Input: part model. Units: mm. Frame: model coordinates. Coordinates: 2 decimals unless noted, no trailing zeros. Loops run counter-clockwise (first coordinate to the right, second up) from the corner with the lowest first, then second, coordinate; pieces in that order, holes last.
Item 1: Section A-A on y = 0. Return loops of the section in (x, z), and give its area (3 significant figures).
Item 2: Contact query for a flat-ended pin moving along its axis: P1, Ø3, axis at x = -9.26, y = 19.87, coming from the +Z side. Output: stop coordinate, or through.
Item 3: Section B-B on x = 5. Return loops of the section in (y, z).
Item 4: Pull-direction query (Y, two-part tool) for faces 1 (the flat face through (-12, 27, 3)), 2 (the cylindrical face through (-21.156, -8.081, 1.521)), 3 (the cylindrical face through (-75.49, -45.72, 1.48)); classes: released by +Y, released by -Y, zero draft, split by the parting line, or undercut.
Item 5: Section C-C on z = 0.8. Give the number of separate pieces and of enclosed holes in the cut face, and give its area (3 significant figures).
Item 6: Ray query, line 1 along X through (y, z) = (89, 2.75); line 2 along Y through (x, z) = (-65, 2.15); line 3 along Y through (x, z) = (-67.5, 0.85). Return the intervals inside material, ascending.
```python
from build123d import *

# Parameters (mm, degrees)
BASE_FLANGE1_DEPTH   = 3
SKETCH2_R            = 15.5
SKETCH2_R_2          = 1.75
CUT_EXTRUDE1_DEPTH   = 131.05864062
M5_CLEARANCE_HOLE1_D = 5.5


# Sheet-metal steps are written as plain solids
with BuildPart() as part:
    # Sketch1 → Base-Flange1 (new body)
    with BuildSketch(Plane.XY):
        with BuildLine():
            Line((-67.5, 102.5), (42.5, 102.5))
            ThreePointArc((42.5, 102.5), (51.338834765, 98.838834765), (55, 90))
            Line((55, 90), (55, -35))
            ThreePointArc((55, -35), (50.606601718, -45.606601718), (40, -50))
            Line((40, -50), (-65, -50))
            ThreePointArc((-65, -50), (-75.606601718, -45.606601718), (-80, -35))
            Line((-80, -35), (-80, 90))
            ThreePointArc((-80, 90), (-76.338834765, 98.838834765), (-67.5, 102.5))
        make_face()
    extrude(amount=BASE_FLANGE1_DEPTH)

    # Sketch2 → Cut-Extrude1 (cut, through all)
    with BuildSketch(Plane.XY.offset(3)):
        Circle(SKETCH2_R)
        with Locations((-19.866547844, -9.263923401)):
            Circle(SKETCH2_R_2)
        with Locations((9.263923401, -19.866547844)):
            Circle(SKETCH2_R_2)
        with Locations((-9.263923401, 19.866547844)):
            Circle(SKETCH2_R_2)
    extrude(amount=-CUT_EXTRUDE1_DEPTH, mode=Mode.SUBTRACT)

    # M5 Clearance Hole1 (through all)
    with Locations(Plane(origin=(0, 0, 0), x_dir=(-1, 0, 0), z_dir=(0, 0, -1))):
        with Locations((-40, -35), (67.5, 90), (65, -35), (-42.5, 90)):
            Hole(M5_CLEARANCE_HOLE1_D / 2)


solid = part.part
```
Results found:
1. outline: (-80, 0) - (-15.5, 0) - (-15.5, 3) - (-80, 3) - close; (15.5, 0) - (55, 0) - (55, 3) - (15.5, 3) - close
1. area: 312 mm2
2. P1: passes through
3. outline: (-50, 0) - (-14.67, 0) - (-14.67, 3) - (-50, 3) - close; (14.67, 0) - (102.5, 0) - (102.5, 3) - (14.67, 3) - close
4. face 1: zero draft
4. face 2: undercut
4. face 3: released by -Y
5. separate pieces: 1
5. enclosed holes: 8
5. area: 19,500 mm2
6. line 1: x = -80 to -70.06, -64.94 to 39.94, 45.06 to 55
6. line 2: y = -50 to -37.75, -32.25 to 88.85, 91.15 to 102.5
6. line 3: y = -49.79 to -36.15, -33.85 to 87.25, 92.75 to 102.5
